The listing builds one solid part. Answer for the finished solid, in the listing's coordinates (mm). A direction names the side the tool comes from. Round coordinates to 2 decimals unless told otherwise and drop trailing zeros. Loops run counter-clockwise (first coordinate to the right, second up) from the corner with the lowest first, then second, coordinate; pieces in that order, holes last. Notation, with made-up numbers: (62, 23) - (73, 23) arc R26 cw to (73, 61) - close; hole circle Ø9 at (43.5, 77.25). An arc over 180 degrees is marked (long way). One line per question, with ' | ' between items. Start each with the question number.
from build123d import *

# Parameters (mm, degrees)
SKETCH_1_W          = 237
SKETCH_1_H          = 145
EXTRUDE_1_DEPTH     = 14
SKETCH_2_R          = 2
SKETCH_2_R_2        = 3
CUT_EXTRUDE_1_DEPTH = 4
SKETCH_3_W          = 31.876725666
SKETCH_3_H          = 70.670873742
CUT_EXTRUDE_2_DEPTH = 8
SKETCH_4_W          = 229
SKETCH_4_H          = 137
CUT_EXTRUDE_3_DEPTH = 0.5
SKETCH_5_W          = 10
SKETCH_5_H          = 6
EXTRUDE_2_DEPTH     = 80


with BuildPart() as part:
    # 草图1 → 凸台-拉伸1 (new body)
    with BuildSketch(Plane(origin=(0, 0, 0), x_dir=(1, 0, 0), z_dir=(0, 1, 0))):
        with Locations((0, 72.5)):
            Rectangle(SKETCH_1_W, SKETCH_1_H)
    extrude(amount=EXTRUDE_1_DEPTH)

    # 草图2 → 切除-拉伸1 (cut)
    with BuildSketch(Plane.XZ):
        with Locations(Location((37.5, -110, 0), (0, 0, 270))):
            Circle(SKETCH_2_R)
        with Locations(Location((-37.5, -110, 0), (0, 0, 270))):
            Circle(SKETCH_2_R)
        with Locations(Location((-37.5, -35, 0), (0, 0, 270))):
            Circle(SKETCH_2_R)
        with Locations(Location((37.5, -35, 0), (0, 0, 270))):
            Circle(SKETCH_2_R)
        with Locations(Location((0, -24, 0), (0, 0, 270))):
            Circle(SKETCH_2_R_2)
    extrude(amount=-CUT_EXTRUDE_1_DEPTH, mode=Mode.SUBTRACT)

    # 草图3 → 切除-拉伸2 (cut)
    with BuildSketch(Plane.XZ):
        with Locations((102.561637167, -51.846473886)):
            Rectangle(SKETCH_3_W, SKETCH_3_H)
    extrude(amount=-CUT_EXTRUDE_2_DEPTH, mode=Mode.SUBTRACT)

    # 草图4 → 切除-拉伸3 (cut)
    with BuildSketch(Plane(origin=(0, 14, 0), x_dir=(1, 0, 0), z_dir=(0, 1, 0))):
        with Locations((0, 72.5)):
            Rectangle(SKETCH_4_W, SKETCH_4_H)
    extrude(amount=-CUT_EXTRUDE_3_DEPTH, mode=Mode.SUBTRACT)

    # 草图5 → 凸台-拉伸2 (add)
    with BuildSketch(Plane(origin=(86.623274334, 0, 0), x_dir=(0, 0, -1), z_dir=(1, 0, 0))):
        with Locations((53.458325759, 3)):
            Rectangle(SKETCH_5_W, SKETCH_5_H)
    extrude(amount=EXTRUDE_2_DEPTH)


solid = part.part
(1) Consider L1, parallel to X at y = 2.75, z = -110; L2, parallel to X at y = 0.95, z = -35; L3, parallel to Z at x = 117, y = 4.5. Determine where each line is inside the solid, lowest interval first.
(2) Find section A-A on x = 20. Write down the section's boundary in (y, z), plus the area to 3 significant figures.
(3) Determine the mould class of faces 4 (the flat face through (-36, 14, -3)), 5 (the flat face through (126, 6, -53)), 6 (the flat face through (0, 4, -24)), 7 (the flat face through (102, 4, -16.511)) for opening direction Y: pulls with the +Y half, pulls with the -Y half, needs draft (parallel to the pull), parting line crosses it, or undercut.
(4) Find section D-D on x = 146.5. Write down the section's boundary in (y, z).
(5) Find section B-B on z = -100. Write down the section's boundary in (x, y), plus the area to 3 significant figures.
(6) A tool of negligible diameter and unlimited length cuts with its end or side. For faces 1 (the cylindrical face through (0, 2, -21)), 2 (the flat face through (102, 4, -87.182)), 3 (the flat face through (-2, 13.5, -73)), from which of +Z, -Z, +X, -X, +Y, -Y can it reach the whole face along a straight path? Write none if from no direction.
(7) Each of these flat-tipped pins is pushed along its axis until it touches: P1, Ø1.5, axis at x = 133, y = 4.5, coming from the -Z side; P2, Ø8, axis at y = 2, z = -92, coming from the +X side; P3, Ø4.5, axis at x = 37.5, z = -110, coming from the +Y side. Where does it stop, or does it pass through?
(8) Find section C-C on y = 10.75. Write down the section's boundary in (x, z).
Answer below:
1) L1: -118.5 to -39.5, -35.5 to 35.5, 39.5 to 118.5 | L2: -118.5 to -39.5, -35.5 to 35.5, 39.5 to 86.62 | L3: -145 to -87.18, -58.46 to -48.46, -16.51 to 0
2) outline: (0, -145) - (14, -145) - (14, -141) - (13.5, -141) - (13.5, -4) - (14, -4) - (14, 0) - (0, 0) - close | area: 1,960 mm2
3) face 4: pulls with the +Y half | face 5: undercut | face 6: pulls with the -Y half | face 7: needs draft
4) outline: (0, -58.46) - (6, -58.46) - (6, -48.46) - (0, -48.46) - close
5) outline: (-118.5, 0) - (118.5, 0) - (118.5, 14) - (114.5, 14) - (114.5, 13.5) - (-114.5, 13.5) - (-114.5, 14) - (-118.5, 14) - close | area: 3,200 mm2
6) face 1: -Y | face 2: +X, -Y | face 3: +Y
7) P1: z = -58.46 | P2: x = 118.5 | P3: y = 13.5
8) outline: (-118.5, -145) - (118.5, -145) - (118.5, 0) - (-118.5, 0) - close
